from build123d import *

# Parameters (mm, degrees)
BOSS_EXTRUDE1_DEPTH = 5
SKETCH2_R           = 6
CUT_EXTRUDE1_DEPTH  = 46.453272709
SKETCH3_R           = 8
CUT_EXTRUDE2_DEPTH  = 4
SKETCH4_R           = 1.75
CUT_EXTRUDE3_DEPTH  = 46.453272709
CUT_EXTRUDE4_DEPTH  = 2
SKETCH6_W           = 42
SKETCH6_H           = 25
BOSS_EXTRUDE2_DEPTH = 9
SKETCH7_R           = 22
CUT_EXTRUDE5_DEPTH  = 47.065171225


with BuildPart() as part:
    # Sketch1 → Boss-Extrude1 (new body)
    with BuildSketch(Plane.XY):
        with BuildLine():
            Line((-21, 40), (21, 40))
            Line((21, 40), (21, 0))
            ThreePointArc((21, 0), (0, -21), (-21, 0))
            Line((-21, 0), (-21, 40))
        make_face()
    extrude(amount=BOSS_EXTRUDE1_DEPTH)

    # Sketch2 → Cut-Extrude1 (cut, through all)
    with BuildSketch(Plane.XY.offset(5)):
        Circle(SKETCH2_R)
    extrude(amount=-CUT_EXTRUDE1_DEPTH, mode=Mode.SUBTRACT)

    # Sketch3 → Cut-Extrude2 (cut)
    with BuildSketch(Plane(origin=(0, 0, 0), x_dir=(-1, 0, 0), z_dir=(0, 0, -1))):
        Circle(SKETCH3_R)
    extrude(amount=-CUT_EXTRUDE2_DEPTH, mode=Mode.SUBTRACT)

    # Sketch4 → Cut-Extrude3 (cut, through all)
    with BuildSketch(Plane(origin=(0, 0, 0), x_dir=(-1, 0, 0), z_dir=(0, 0, -1))):
        with Locations((-11, 11)):
            Circle(SKETCH4_R)
        with Locations(Location((-11, -11, 0), (0, 0, 180))):
            Circle(SKETCH4_R)
        with Locations((11, -11)):
            Circle(SKETCH4_R)
        with Locations(Location((11, 11, 0), (0, 0, 180))):
            Circle(SKETCH4_R)
    extrude(amount=-CUT_EXTRUDE3_DEPTH, mode=Mode.SUBTRACT)

    # Sketch5 → Cut-Extrude4 (cut)
    with BuildSketch(Plane(origin=(0, 0, 0), x_dir=(-1, 0, 0), z_dir=(0, 0, -1))):
        Polygon((-11, 14.290896534), (-13.85, 12.645448267), (-13.85, 9.354551733), (-11, 7.709103466), (-8.15, 9.354551733), (-8.15, 12.645448267), align=None)
        Polygon((-8.15, -12.645448267), (-11, -14.290896534), (-13.85, -12.645448267), (-13.85, -9.354551733), (-11, -7.709103466), (-8.15, -9.354551733), align=None)
        Polygon((11, -14.290896534), (13.85, -12.645448267), (13.85, -9.354551733), (11, -7.709103466), (8.15, -9.354551733), (8.15, -12.645448267), align=None)
        Polygon((8.15, 12.645448267), (11, 14.290896534), (13.85, 12.645448267), (13.85, 9.354551733), (11, 7.709103466), (8.15, 9.354551733), align=None)
    extrude(amount=-CUT_EXTRUDE4_DEPTH, mode=Mode.SUBTRACT)

    # Sketch6 → Boss-Extrude2 (add)
    with BuildSketch(Plane(origin=(0, 0, 0), x_dir=(-1, 0, 0), z_dir=(0, 0, -1))):
        with Locations((0, 27.5)):
            Rectangle(SKETCH6_W, SKETCH6_H)
    extrude(amount=BOSS_EXTRUDE2_DEPTH)

    # Sketch7 → Cut-Extrude5 (cut, through all)
    with BuildSketch(Plane(origin=(0, 0, 0), x_dir=(-1, 0, 0), z_dir=(0, 0, -1))):
        Circle(SKETCH7_R)
    extrude(amount=CUT_EXTRUDE5_DEPTH, mode=Mode.SUBTRACT)


solid = part.part
CAD build for the part. Positions are in the model's coordinates, mm. A direction names the side the tool comes from. Coordinates: 2 decimals unless noted, no trailing zeros. Loops run counter-clockwise (first coordinate to the right, second up) from the corner with the lowest first, then second, coordinate; pieces in that order, holes last. Notation, with made-up numbers: (-19.75, -5.5) - (5.25, -5.5) arc R13 ccw to (5.25, 19.5) - close; hole circle Ø6 at (-29, 67.25). An arc over 180 degrees is marked (long way). Use one line per item in the form item = value. Start each with the question number.
1) Flat gauge pins, fed straight in: pin 1 (4.5 mm diameter, centred on x = -10.5, y = -11, fed in from -Z); pin 2 (4 mm diameter, centred on x = 19.5, z = -4.5, fed in from -Y); pin 3 (13 mm diameter, centred on x = 3.5, y = -0.5, fed in from -Z). Where does each tip first touch, or does it go through?
2) Band-saw the part on A-A (y = 11). Give the cut face in (x, z).
3) Drill centre lines: L1, parallel to Y at x = 11, z = 0.25; L2, parallel to Y at x = 0, z = 3; L3, parallel to Y at x = 11, z = 4.4. Where is each one in solid material? Low to high. Write a range as from..to.
4) Band-saw the part on D-D (z = -1.5). Give the cut face in (x, y), and give its area (3 significant figures).
5) Band-saw the part on C-C (y = -4.5). Give the cut face in (x, z).
6) Band-saw the part on B-B (x = 1.5). Give the cut face in (y, z), and give its area (3 significant figures).
7) Two-plate mould, pull along X, no slides. Class faces 3 (the face through (8.15, 11, 1)), 4 (the face through (0, -21, 2)), 5 (the face through (-19, 15, -4)): +X half, -X half, draft (parallel to the pull), parting line (faces both ways), or undercut.
8) Tool access for faces 1 (the face through (12.405, 13.48, 0.986)), 2 (the face through (-11.9, -9.5, 3.5)): list every direction of +Z, -Z, +X, -X, +Y, -Y with a clear straight run to the whole face (end or side of a thin tool).
Check values:
q1.pin_1 = 2
q1.pin_2 = 15
q1.pin_3 = 0
q2.outline = (-21, 0) - (-13.85, 0) - (-13.85, 2) - (-12.75, 2) - (-12.75, 5) - (-21, 5) - close; (-9.25, 2) - (-8.15, 2) - (-8.15, 0) - (8.15, 0) - (8.15, 2) - (9.25, 2) - (9.25, 5) - (-9.25, 5) - close; (12.75, 2) - (13.85, 2) - (13.85, 0) - (21, 0) - (21, 5) - (12.75, 5) - close
q3.L1 = -17.89..-14.29, -7.71..7.71, 14.29..40
q3.L2 = -21..-8, 8..40
q3.L3 = -17.89..-12.75, -9.25..9.25, 12.75..40
q4.outline = (-21, 15) - (-16.09, 15) arc R22 cw to (16.09, 15) - (21, 15) - (21, 40) - (-21, 40) - close
q4.area = 894 mm2
q5.outline = (-20.51, 0) - (-6.61, 0) - (-6.61, 4) - (-3.97, 4) - (-3.97, 5) - (-20.51, 5) - close; (3.97, 4) - (6.61, 4) - (6.61, 0) - (20.51, 0) - (20.51, 5) - (3.97, 5) - close
q6.outline = (-20.95, 0) - (-7.86, 0) - (-7.86, 4) - (-5.81, 4) - (-5.81, 5) - (-20.95, 5) - close; (5.81, 4) - (7.86, 4) - (7.86, 0) - (21.95, 0) - (21.95, -9) - (40, -9) - (40, 5) - (5.81, 5) - close
q6.area = 393 mm2
q7.face_3 = undercut
q7.face_4 = parting line
q7.face_5 = draft
q8.face_1 = -Z
q8.face_2 = +Z, -Z
